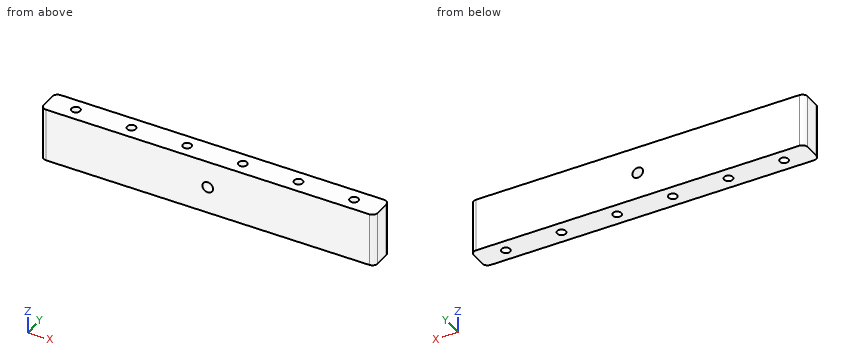
from build123d import *

# Parameters (mm, degrees)
SKETCH1_W               = 156
SKETCH1_H               = 25
SKETCH1_R               = 2.5
BOSS_EXTRUDE1_DEPTH     = 6
FILLET1_R               = 2.5
SKETCH2_R               = 2
CUT_EXTRUDE1_DEPTH      = 10
LPATTERN1_COUNT         = 6
LPATTERN1_PITCH         = 26
MIRROR1_COPY_1_SKETCH_R = 2
MIRROR1_COPY_1_DEPTH    = 10
MIRROR1_COPY_2_SKETCH_R = 2
MIRROR1_COPY_2_DEPTH    = 10
MIRROR1_COPY_3_SKETCH_R = 2
MIRROR1_COPY_3_DEPTH    = 10
MIRROR1_COPY_4_SKETCH_R = 2
MIRROR1_COPY_4_DEPTH    = 10
MIRROR1_COPY_5_SKETCH_R = 2
MIRROR1_COPY_5_DEPTH    = 10


with BuildPart() as part:
    # Sketch1 → Boss-Extrude1 (new, symmetric)
    with BuildSketch(Plane(origin=(0, 0, 0), x_dir=(1, 0, 0), z_dir=(0, 1, 0))):
        Rectangle(SKETCH1_W, SKETCH1_H)
        with Locations(Location((0, 0, 0), (0, 0, 270))):
            Circle(SKETCH1_R, mode=Mode.SUBTRACT)
    extrude(amount=BOSS_EXTRUDE1_DEPTH, both=True)

    # Fillet1
    fillet1_edges = [part.edges().sort_by_distance(p)[0] for p in [
        (-78, 6, 0),
        (78, 6, 0),
        (-78, -6, 0),
        (78, -6, 0),
    ]]
    fillet(fillet1_edges, radius=FILLET1_R)

    # Sketch2 → Cut-Extrude1 (cut)
    with BuildSketch(Plane.XY.offset(12.5)):
        with Locations((-65, 0)):
            Circle(SKETCH2_R)
    cut_extrude1 = extrude(amount=-CUT_EXTRUDE1_DEPTH, mode=Mode.SUBTRACT)

    # LPattern1: Cut-Extrude1 ×6
    with Locations(*[(i * LPATTERN1_PITCH, 0, 0) for i in range(1, LPATTERN1_COUNT)]):
        add(cut_extrude1, mode=Mode.SUBTRACT)

    # Mirror1: Cut-Extrude1 across plane
    add(cut_extrude1.mirror(Plane.XY), mode=Mode.SUBTRACT)

    # Mirror1 copy 1 sketch → Mirror1 copy 1 (cut)
    with BuildSketch(Plane(origin=(26, 0, -12.5), x_dir=(1, 0, 0), z_dir=(0, 0, -1))):
        with Locations((-65, 0)):
            Circle(MIRROR1_COPY_1_SKETCH_R)
    extrude(amount=-MIRROR1_COPY_1_DEPTH, mode=Mode.SUBTRACT)

    # Mirror1 copy 2 sketch → Mirror1 copy 2 (cut)
    with BuildSketch(Plane(origin=(52, 0, -12.5), x_dir=(1, 0, 0), z_dir=(0, 0, -1))):
        with Locations((-65, 0)):
            Circle(MIRROR1_COPY_2_SKETCH_R)
    extrude(amount=-MIRROR1_COPY_2_DEPTH, mode=Mode.SUBTRACT)

    # Mirror1 copy 3 sketch → Mirror1 copy 3 (cut)
    with BuildSketch(Plane(origin=(78, 0, -12.5), x_dir=(1, 0, 0), z_dir=(0, 0, -1))):
        with Locations((-65, 0)):
            Circle(MIRROR1_COPY_3_SKETCH_R)
    extrude(amount=-MIRROR1_COPY_3_DEPTH, mode=Mode.SUBTRACT)

    # Mirror1 copy 4 sketch → Mirror1 copy 4 (cut)
    with BuildSketch(Plane(origin=(104, 0, -12.5), x_dir=(1, 0, 0), z_dir=(0, 0, -1))):
        with Locations((-65, 0)):
            Circle(MIRROR1_COPY_4_SKETCH_R)
    extrude(amount=-MIRROR1_COPY_4_DEPTH, mode=Mode.SUBTRACT)

    # Mirror1 copy 5 sketch → Mirror1 copy 5 (cut)
    with BuildSketch(Plane(origin=(130, 0, -12.5), x_dir=(1, 0, 0), z_dir=(0, 0, -1))):
        with Locations((-65, 0)):
            Circle(MIRROR1_COPY_5_SKETCH_R)
    extrude(amount=-MIRROR1_COPY_5_DEPTH, mode=Mode.SUBTRACT)


solid = part.part
Geometry check sheet. Reference: the model listing, model coordinates, mm. Round coordinates to 2 decimals unless told otherwise and drop trailing zeros. Order: outer loops, then holes, each group sorted by start corner. A loop starts at its lowest first (then second) coordinate and runs counter-clockwise, first axis right, second up. Notation, with made-up numbers: (37.25, -13.75) -> (61.25, -13.75) arc R27 ccw to (61.25, 11.25) -> close; hole circle Ø10 at (68, 85.5). An arc over 180 degrees is marked (long way). Use one line per item in the form item = value.
1. Cross-section at B-B, the plane x = 0. Enter the section's corners in (y, z).
Working result:
outline = (-6, -12.5) -> (6, -12.5) -> (6, -2.5) -> (-6, -2.5) -> close; (-6, 2.5) -> (6, 2.5) -> (6, 12.5) -> (-6, 12.5) -> close
2. Scan lines: line 1 along Y through (x, z) = (-13, 6); line 2 along X through (y, z) = (4.5, 0.5); line 3 along X through (y, z) = (-5.25, 3.75). Record each from-to range of solid material in increasing order. Write a range as from..to.
Working result:
line_1 = -6..-2, 2..6
line_2 = -77.79..-2.45, 2.45..77.79
line_3 = -77.29..77.29
3. Cross-section at C-C, the plane x = -39. Enter the section's corners in (y, z).
Working result:
outline = (-6, -12.5) -> (-2, -12.5) -> (-2, -2.5) -> (2, -2.5) -> (2, -12.5) -> (6, -12.5) -> (6, 12.5) -> (2, 12.5) -> (2, 2.5) -> (-2, 2.5) -> (-2, 12.5) -> (-6, 12.5) -> close
4. Cross-section at A-A, the plane z = -10.5. Enter the section's corners in (x, y), plus the area to 3 significant figures.
Working result:
outline = (-78, -3.5) arc R2.5 ccw to (-75.5, -6) -> (75.5, -6) arc R2.5 ccw to (78, -3.5) -> (78, 3.5) arc R2.5 ccw to (75.5, 6) -> (-75.5, 6) arc R2.5 ccw to (-78, 3.5) -> close; hole circle Ø4 at (-65, 0); hole circle Ø4 at (-39, 0); hole circle Ø4 at (-13, 0); hole circle Ø4 at (13, 0); hole circle Ø4 at (39, 0); hole circle Ø4 at (65, 0)
area = 1,790 mm^2
5. Go/stop test with flat-tipped pins: pin 1 (1.2 mm diameter, centred on x = 65, y = 0.5, fed in from -Z); pin 2 (1 mm diameter, centred on y = -4.5, z = -8, fed in from +X). Record where each tip stops, or that it passes through.
Working result:
pin_1 = -2.5
pin_2 = 77.95
